```python
from build123d import *

# Parameters (mm, degrees)
SKETCH1_W           = 50
SKETCH1_H           = 34
BOSS_EXTRUDE1_DEPTH = 60
CUT_EXTRUDE1_DEPTH  = 68.186308129
SKETCH3_R           = 2.25
CUT_EXTRUDE2_DEPTH  = 74.35529974
CUT_EXTRUDE3_DEPTH  = 24.8
CHAMFER1_SIZE       = 1
CHAMFER1_SIZE_2     = 1.220120443
SKETCH5_R           = 7
BOSS_EXTRUDE2_DEPTH = 14
SKETCH6_R           = 7
SKETCH6_R_2         = 4.15
BOSS_EXTRUDE3_DEPTH = 20
CHAMFER2_SIZE       = 10
CHAMFER2_SIZE2      = 0.174550649
CHAMFER4_SIZE       = 10


with BuildPart() as part:
    # Sketch1 → Boss-Extrude1 (new body)
    with BuildSketch(Plane(origin=(0, 0, 0), x_dir=(1, 0, 0), z_dir=(0, 1, 0))):
        Rectangle(SKETCH1_W, SKETCH1_H)
    extrude(amount=BOSS_EXTRUDE1_DEPTH)

    # Sketch2 → Cut-Extrude1 (cut, through all)
    with BuildSketch(Plane(origin=(0, 60, 0), x_dir=(1, 0, 0), z_dir=(0, 1, 0))):
        with BuildLine():
            Line((-3.75, 3.5), (-7, -2.8))
            Line((-7, -2.8), (-7, -9.8))
            Line((-7, -9.8), (-15.5, -9.8))
            Line((-15.5, -9.8), (-15.5, -14))
            Line((-15.5, -14), (15.5, -14))
            Line((15.5, -14), (15.5, -9.8))
            Line((15.5, -9.8), (7, -9.8))
            Line((7, -9.8), (7, -2.8))
            Line((7, -2.8), (3.75, 3.5))
            ThreePointArc((3.75, 3.5), (0, 14.75), (-3.75, 3.5))
        make_face()
    extrude(amount=-CUT_EXTRUDE1_DEPTH, mode=Mode.SUBTRACT)

    # Sketch3 → Cut-Extrude2 (cut, through all)
    with BuildSketch(Plane.XY.offset(17)):
        with Locations((-11, 50)):
            Circle(SKETCH3_R)
        with Locations((11, 50)):
            Circle(SKETCH3_R)
    extrude(amount=-CUT_EXTRUDE2_DEPTH, mode=Mode.SUBTRACT)

    # Sketch4 → Cut-Extrude3 (cut)
    with BuildSketch(Plane(origin=(0, 0, -17), x_dir=(-1, 0, 0), z_dir=(0, 0, -1))):
        Polygon((14.75, 52.165063509), (11, 54.330127019), (7.25, 52.165063509), (7.25, 47.834936491), (11, 45.669872981), (14.75, 47.834936491), align=None)
        Polygon((-7.25, 47.834936491), (-7.25, 52.165063509), (-11, 54.330127019), (-14.75, 52.165063509), (-14.75, 47.834936491), (-11, 45.669872981), align=None)
    extrude(amount=-CUT_EXTRUDE3_DEPTH, mode=Mode.SUBTRACT)

    # Chamfer1
    # the kernel refuses this chamfer: 1.220120443, 1 mm, written as the material it takes off along each edge
    with BuildSketch(Plane(origin=(-7, 62.571682988, 9.8), x_dir=(-1, 0, 0), z_dir=(0, -1, 0)), Plane(origin=(7, 62.571682988, 9.8), x_dir=(0, 0, -1), z_dir=(0, -1, 0))) as chamfer1_piece_1:
        Polygon((CHAMFER1_SIZE, 0), (0, CHAMFER1_SIZE), (0, 0), align=None)
    extrude(amount=65.143365976, mode=Mode.SUBTRACT)
    with BuildSketch(Plane(origin=(-3.75, 63.150527813, -3.5), x_dir=(-0.45846324589157744, 0, 0.8887133689590581), z_dir=(0, -1, 0))) as chamfer1_piece_2:
        with BuildLine():
            Line((CHAMFER1_SIZE_2, 0), (-0.278286757, 1.065574765))
            ThreePointArc((-0.278286757, 1.065574765), (-0.120412167, 0.557139368), (0, 0))
            Line((0, 0), (CHAMFER1_SIZE_2, 0))
        make_face()
    extrude(amount=66.301055626, mode=Mode.SUBTRACT)
    with BuildSketch(Plane(origin=(3.75, 63.795705698, -3.5), x_dir=(0.7235959376340886, 0, -0.6902238180760238), z_dir=(0, -1, 0))) as chamfer1_piece_3:
        with BuildLine():
            Line((1.475268649, 0), (-CHAMFER1_SIZE * 0.281668992416, CHAMFER1_SIZE * 0.959511635527))
            Line((-CHAMFER1_SIZE * 0.281668992416, CHAMFER1_SIZE * 0.959511635527), (0, 0))
            ThreePointArc((0, 0), (0.759242358, 0.043643641), (1.475268649, 0))
        make_face()
    extrude(amount=67.591411396, mode=Mode.SUBTRACT)

    # Sketch5 → Boss-Extrude2 (add)
    with BuildSketch(Plane(origin=(0, 0, -17), x_dir=(-1, 0, 0), z_dir=(0, 0, -1))):
        with Locations(Location((0, 25, 0), (0, 0, 180))):
            Circle(SKETCH5_R)
    extrude(amount=BOSS_EXTRUDE2_DEPTH)

    # Sketch6 → Boss-Extrude3 (add)
    with BuildSketch(Plane(origin=(0, 0, -31), x_dir=(-1, 0, 0), z_dir=(0, 0, -1))):
        with Locations(Location((0, 25, 0), (0, 0, 180))):
            Circle(SKETCH6_R)
        with Locations((0, 25)):
            Circle(SKETCH6_R_2, mode=Mode.SUBTRACT)
    extrude(amount=BOSS_EXTRUDE3_DEPTH)

    # Chamfer2
    chamfer2_edges = [part.edges().sort_by_distance(p)[0] for p in [
        (4.15, 25, -31),
    ]]
    chamfer2_side = [part.faces().sort_by_distance(p)[0] for p in [
        (4.15, 25, -41),
    ]]
    chamfer(chamfer2_edges, length=CHAMFER2_SIZE, length2=CHAMFER2_SIZE2, reference=chamfer2_side[0])

    # Chamfer4
    chamfer4_edges = [part.edges().sort_by_distance(p)[0] for p in [
        (-7, 25, -17),
    ]]
    chamfer(chamfer4_edges, length=CHAMFER4_SIZE)


solid = part.part
```
Model file for the job. Use its own axes, mm. A direction names the side the tool comes from. Round coordinates to 2 decimals unless told otherwise and drop trailing zeros. Write each loop counter-clockwise with the first axis right and the second up, starting at its lowest first coordinate (ties: lowest second). Pieces come first, ordered by that corner, then holes. Notation, with made-up numbers: (66, -28) -> (78, -28) arc R26 ccw to (78, 9) -> close; hole circle Ø2 at (2.5, 87.25). An arc over 180 degrees is marked (long way). Answer as CSV lines item,"result".
1. Slice it at A-A, the plane z = 4. List the corners of the cut face in (x, y), plus the area to 3 significant figures.
Resolved:
outline,"(-25, 0) -> (-7, 0) -> (-7, 60) -> (-25, 60) -> close; (7, 0) -> (25, 0) -> (25, 60) -> (7, 60) -> close; hole (-14.75, 47.83) -> (-11, 45.67) -> (-7.25, 47.83) -> (-7.25, 52.17) -> (-11, 54.33) -> (-14.75, 52.17) -> close; hole (7.25, 47.83) -> (11, 45.67) -> (14.75, 47.83) -> (14.75, 52.17) -> (11, 54.33) -> (7.25, 52.17) -> close"
area,"2,060 mm²"
2. Slice it at D-D, the plane z = -23. List the corners of the cut face in (x, y), plus the area to 3 significant figures.
Resolved:
outline,"circle Ø22 at (0, 25)"
area,"380 mm²"
3. Tool access for faces 1 (the face through (10.71, 52.23, 15.52)), 2 (the face through (-12.901, 53.232, -4.774)), 3 (the face through (0, 30, 14)): list every direction of +Z, -Z, +X, -X, +Y, -Y with a clear straight run to the whole face (end or side of a thin tool).
Resolved:
face 1,"+Z, -Z"
face 2,"-Z"
face 3,"+Y, -Y"
4. Slice it at B-B, the plane z = -8.5. List the corners of the cut face in (x, y), plus the area to 3 significant figures.
Resolved:
outline,"(-25, 0) -> (-6.25, 0) -> (-6.25, 60) -> (-25, 60) -> close; (6.25, 0) -> (25, 0) -> (25, 60) -> (6.25, 60) -> close; hole (-14.75, 47.83) -> (-11, 45.67) -> (-7.25, 47.83) -> (-7.25, 52.17) -> (-11, 54.33) -> (-14.75, 52.17) -> close; hole (7.25, 47.83) -> (11, 45.67) -> (14.75, 47.83) -> (14.75, 52.17) -> (11, 54.33) -> (7.25, 52.17) -> close"
area,"2,150 mm²"
5. Slice it at C-C, the plane x = -20.5. List the corners of the cut face in (y, z), plus the area to 3 significant figures.
Resolved:
outline,"(0, -17) -> (60, -17) -> (60, 17) -> (0, 17) -> close"
area,"2,040 mm²"
6. Mould opens along X. For faces 4 (the face through (-1.653, 32.444, -26.374)), 5 (the face through (-12.85, 46.74, -4.77)), 6 (the face through (25, 30, 0)), 7 (the face through (7.25, 50, -5)) say: +X half, -X half, draft (parallel to the pull), parting line (faces both ways), or undercut.
Resolved:
face 4,"parting line"
face 5,"undercut"
face 6,"+X half"
face 7,"undercut"
7. Drill centre lines: line 1 (Z direction, x = -11.5, y = 3.5); line 2 (Z direction, x = 0, y = 19); line 3 (Y direction, x = 11, z = 15.65). Where is each one in solid material? Low to high.
Resolved:
line 1,"-17 to 9.8, 14 to 17"
line 2,"-51 to -14.75, 14 to 17"
line 3,"0 to 47.75, 52.25 to 60"
8. Pin check, flat tips, straight feed: pin 1 Ø3.5 at (x, y) = (11, 50) entering from -Z; pin 2 Ø4 at (x, y) = (9.5, 50) entering from -Z; pin 3 Ø1.5 at (x, y) = (9.5, 29) entering from -Z; pin 4 Ø8 at (x, y) = (-11, 48) entering from -Z. Stop position of each tip, or through.
Resolved:
pin 1,"through"
pin 2,"z = 7.8"
pin 3,"z = -24.44"
pin 4,"z = -17"
